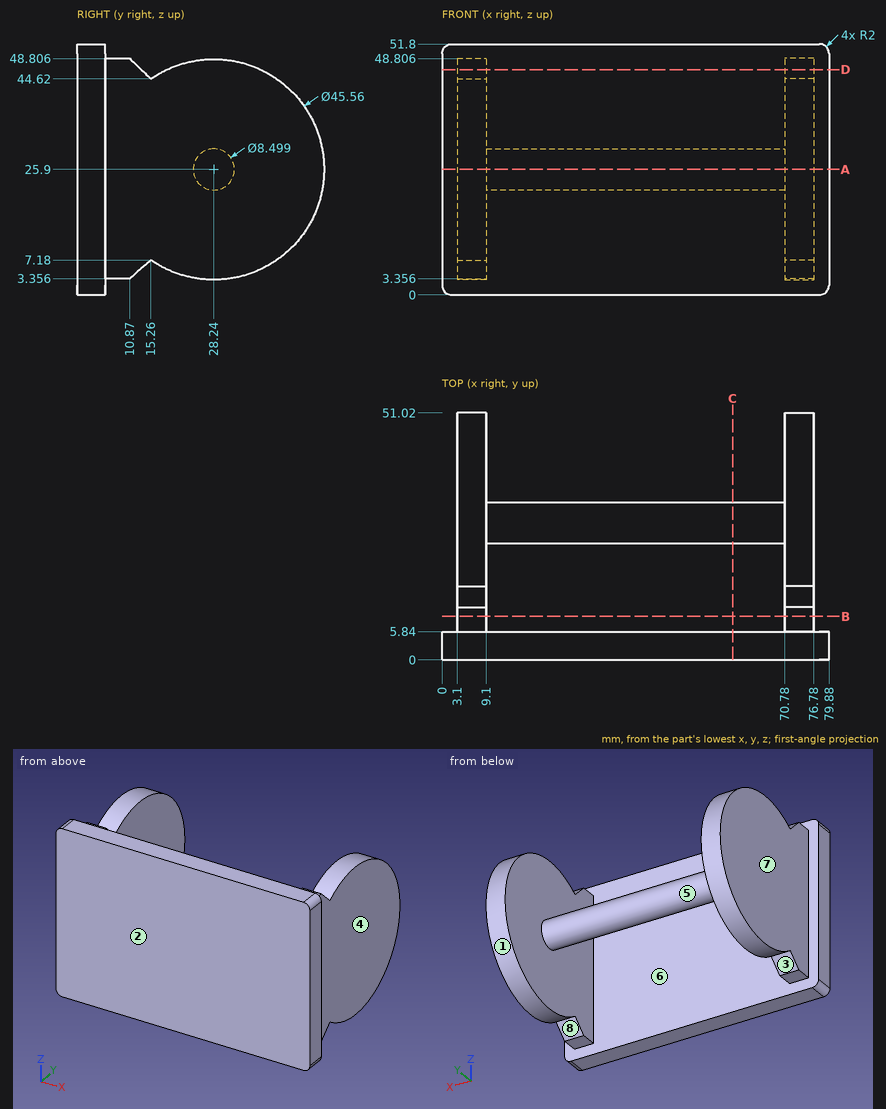
Input: dimensioned drawing with shaded views. Units: mm. Origin: part minimum x, y, z. A direction names the side the tool comes from. Coordinates: 2 decimals unless noted, no trailing zeros. Loops run counter-clockwise (first coordinate to the right, second up) from the corner with the lowest first, then second, coordinate; pieces in that order, holes last. Notation, with made-up numbers: M -13.5,72.5 L 32.5,72.5 A5 ccw 32.5,76.5 Z; hole C 23,29.5 d1. An arc over 180 degrees is marked long. Use a Markdown table: item, result. Add a question column.
1) Set-up query: the marked faces 1, 2, 3, 4 and 5. Return all of +Z, -Z, +X, -X, +Y, -Y with unobstructed straight access to the full face (end or side cutting, diameter ignored); none if empty.
2) Line query: L1, parallel to X at y = 33, z = 30.5; L2, parallel to Y at x = 26, z = 31; L3, parallel to Y at x = 18.5, z = 27 (1 decimal). Output: solid intervals per line, ascending. Write a range as from..to.
3) Pin query (flat end, axial travel): P1, Ø22.5, axis at y = 19, z = 16, coming from the -X side; P2, Ø5.5, axis at x = 73, y = 9, coming from the +Z side; P3, Ø15.5, axis at x = 24, z = 15.5, coming from the +Y side. Return the tip coordinate at first contact, or that it passes through.
4) Section B-B, the plane y = 9. Return the cut outline in (x, z).
5) Section A-A, the plane z = 25.9. Return the cut outline in (x, y).
6) Section D-D, the plane z = 46.5. Return the cut outline in (x, y) (1 decimal).
7) Draft query along X for the marked faces 6, 7 and 8. Return one class per face: +X half, -X half, draft (parallel to the pull), parting line (faces both ways), or undercut.
8) Section C-C, the plane x = 60. Return the cut outline in (y, z), plus the area to 3 significant figures.
Answer below:
| question | item | result |
|---|---|---|
| 1 | face 1 | +X, -X |
| 1 | face 2 | +Z, -Z, +X, -X, -Y |
| 1 | face 3 | -Z, +X, -X |
| 1 | face 4 | +Z, -Z, +X, +Y |
| 1 | face 5 | none |
| 2 | L1 | 3.1..9.1, 70.78..76.78 |
| 2 | L2 | 0..5.84 |
| 2 | L3 | 0..5.8, 24.1..32.3 |
| 3 | P1 | x = 3.1 |
| 3 | P2 | z = 48.81 |
| 3 | P3 | y = 31.56 |
| 4 | outline | M 3.1,3.36 L 9.1,3.36 L 9.1,48.81 L 3.1,48.81 Z; M 70.78,3.36 L 76.78,3.36 L 76.78,48.81 L 70.78,48.81 Z |
| 5 | outline | M 0,0 L 79.88,0 L 79.88,5.84 L 76.78,5.84 L 76.78,51.02 L 70.78,51.02 L 70.78,32.49 L 9.1,32.49 L 9.1,51.02 L 3.1,51.02 L 3.1,5.84 L 0,5.84 Z; hole M 9.1,5.84 L 70.78,5.84 L 70.78,23.99 L 9.1,23.99 Z |
| 6 | outline | M 0,0 L 79.9,0 L 79.9,5.8 L 76.8,5.8 L 76.8,13.3 L 70.8,13.3 L 70.8,5.8 L 9.1,5.8 L 9.1,13.3 L 3.1,13.3 L 3.1,5.8 L 0,5.8 Z; M 3.1,18.5 L 9.1,18.5 L 9.1,38 L 3.1,38 Z; M 70.8,18.5 L 76.8,18.5 L 76.8,38 L 70.8,38 Z |
| 7 | face 6 | undercut |
| 7 | face 7 | -X half |
| 7 | face 8 | draft |
| 8 | outline | M 0,0 L 5.84,0 L 5.84,51.8 L 0,51.8 Z; C 28.24,25.9 d8.5 |
| 8 | area | 359 mm2 |
